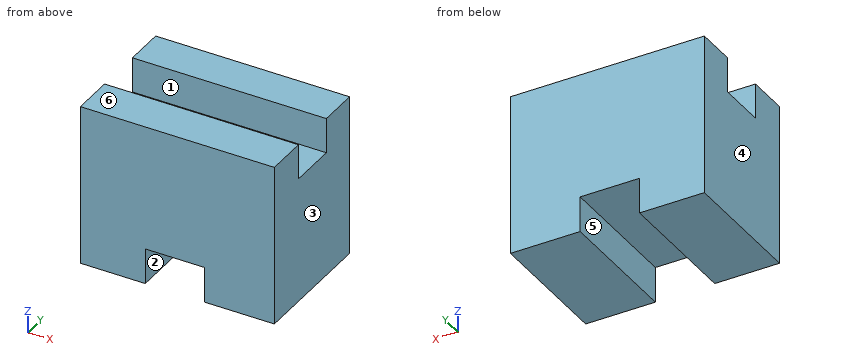
from build123d import *

# Parameters (mm, degrees)
F0_W     = 25.5834441632
F0_H     = 31.7076668143
F1_DEPTH = 38.1
F2_W     = 9.4826659188
F2_H     = 6.9144461304
F3_DEPTH = 38.1
F4_W     = 11.6557758301
F4_H     = 7.0132222027
F5_DEPTH = 38.1


with BuildPart() as f1:
    # F0 (on Right) → F1 (new body)
    with BuildSketch(Plane.YZ):
        with Locations((12.7917220816, 15.8538334072)):
            Rectangle(F0_W, F0_H)
    extrude(amount=F1_DEPTH)

    # F2 (on face) → F3 (cut)
    with BuildSketch(Plane.YZ.offset(38.1)):
        with Locations((12.9398894496, 28.2504437491)):
            Rectangle(F2_W, F2_H)
    extrude(amount=-F3_DEPTH, mode=Mode.SUBTRACT)

    # F4 (on face) → F5 (cut)
    with BuildSketch(Plane.XZ):
        with Locations((18.5702228919, 3.5066111013)):
            Rectangle(F4_W, F4_H)
    extrude(amount=-F5_DEPTH, mode=Mode.SUBTRACT)


solid = f1.part
Could you check a few things on this model? Use its own coordinates, in mm. Face numbers are marked on the shaded views. A direction names the side the tool comes from. Coordinates: 2 decimals unless noted, no trailing zeros. Order: outer loops, then holes, each group sorted by start corner. A loop starts at its lowest first (then second) coordinate and runs counter-clockwise, first axis right, second up.
Q1. Thinking about a two-plate mould opening in X: for the marked faces 4, 5 and 6, which applies, released by +X, released by -X, zero draft, split by the parting line, or undercut?
Q2. Suppose I cut it at C-C on x = 4.5. Please give me the cut outline in (y, z), and give its area (3 significant figures).
Q3. Will these pins go through, and if not, where does the flat tip stop? pin 1 (3 mm diameter, centred on x = 8, y = 11, fed in from +Z); pin 2 (6 mm diameter, centred on x = 20.5, y = 12, fed in from -Z).
Q4. Suppose I cut it at A-A on z = 28.5. Please give me the cut outline in (x, y).
Q5. Please list where these lines run through material, in increasing order: L1, parallel to Y at x = 24.5, z = 26.5; L2, parallel to X at y = 15.5, z = 5; L3, parallel to Z at x = 14, y = 16.25.
Q6. Suppose I cut it at B-B on y = 12.5. Please give me the cut outline in (x, z).
Q7. Which directions (+Z, -Z, +X, -X, +Y, -Y) give clear straight access to the entire face, cutting with the end or side of a thin tool? Please do the marked faces 1, 2 and 3.
Answer:
1. face 4: released by -X
1. face 5: undercut
1. face 6: zero draft
2. outline: (0, 0) - (25.58, 0) - (25.58, 31.71) - (17.68, 31.71) - (17.68, 24.79) - (8.2, 24.79) - (8.2, 31.71) - (0, 31.71) - close
2. area: 746 mm2
3. pin 1: stops at z = 24.79
3. pin 2: stops at z = 7.01
4. outline: (0, 0) - (38.1, 0) - (38.1, 8.2) - (0, 8.2) - close; (0, 17.68) - (38.1, 17.68) - (38.1, 25.58) - (0, 25.58) - close
5. L1: y = 0 to 8.2, 17.68 to 25.58
5. L2: x = 0 to 12.74, 24.4 to 38.1
5. L3: z = 7.01 to 24.79
6. outline: (0, 0) - (12.74, 0) - (12.74, 7.01) - (24.4, 7.01) - (24.4, 0) - (38.1, 0) - (38.1, 24.79) - (0, 24.79) - close
7. face 1: +Z, +X, -X
7. face 2: -Z, +Y, -Y
7. face 3: +Z, -Z, +X, +Y, -Y
